```python
from build123d import *

# Parameters (mm, degrees)
EXTRUDE_1_DEPTH     = 9
EXTRUDE_2_DEPTH     = 13
SKETCH_5_R          = 4.25
CUT_EXTRUDE_1_DEPTH = 7


with BuildPart() as part:
    # Эскиз1 → Повернуть1 (revolve)
    with BuildSketch(Plane.XY, mode=Mode.PRIVATE) as revolve_1_sk:
        Polygon((0, 0), (-30, 0), (-30, 6), (-17, 6), (-16, 20), (-12, 20), (-12, 22), (-8, 26), (-8, 29), (-8, 38), (-8, 186), (-6, 188), (0, 188), align=None)
    revolve(revolve_1_sk.sketch.rotate(Axis((0, 0, 0), (0, 1, 0)), 180), axis=Axis((0, 0, 0), (0, 1, 0)))  # turned: the seam where the file's is

    # Эскиз2 → Бобышка-Вытянуть1 (add)
    with BuildSketch(Plane(origin=(0, 29, 0), x_dir=(1, 0, 0), z_dir=(0, 1, 0))):
        Polygon((0, 13.856406461), (-12, 6.92820323), (-12, -6.92820323), (0, -13.856406461), (12, -6.92820323), (12, 6.92820323), align=None)
    extrude(amount=EXTRUDE_1_DEPTH)

    # Эскиз3 → Бобышка-Вытянуть2 (add)
    with BuildSketch(Plane(origin=(0, 112, 0), x_dir=(1, 0, 0), z_dir=(0, 1, 0))):
        Polygon((12, 6.92820323), (0, 13.856406461), (-12, 6.92820323), (-12, -6.92820323), (0, -13.856406461), (12, -6.92820323), align=None)
    extrude(amount=EXTRUDE_2_DEPTH)

    # Эскиз4 → Вырез-Повернуть2 (revolve, cut)
    with BuildSketch(Plane.XY, mode=Mode.PRIVATE) as cut_revolve_2_sk:
        Polygon((-23.258330249, 125), (-12, 125), (-23.258330249, 118.5), align=None)
        Polygon((-23.258330249, 112), (-23.258330249, 118.5), (-12, 112), align=None)
        Polygon((-19.794228634, 38), (-19.794228634, 33.5), (-12, 38), align=None)
        Polygon((-19.794228634, 33.5), (-19.794228634, 29), (-12, 29), align=None)
    revolve(cut_revolve_2_sk.sketch.rotate(Axis((0, 188, 0), (0, -1, 0)), 180), axis=Axis((0, 188, 0), (0, -1, 0)), mode=Mode.SUBTRACT)  # turned: the seam where the file's is

    # Эскиз5 → Вырез-Вытянуть1 (cut, through all)
    with BuildSketch(Plane(origin=(0, 6, 0), x_dir=(1, 0, 0), z_dir=(0, 1, 0))):
        with Locations(Location((-23.75, 0, 0), (0, 0, 180))):  # turned: the seam where the file's is
            Circle(SKETCH_5_R)
        with Locations(Location((23.75, 0, 0), (0, 0, 180))):  # turned: the seam where the file's is
            Circle(SKETCH_5_R)
    extrude(amount=-CUT_EXTRUDE_1_DEPTH, mode=Mode.SUBTRACT)


solid = part.part
```
The model under review builds one solid part; all positions refer to its coordinate system, in mm. A direction names the side the tool comes from. Give positions to 0.01 mm unless a question says otherwise; leave off trailing zeros. Loops run counter-clockwise (first coordinate to the right, second up) from the corner with the lowest first, then second, coordinate; pieces in that order, holes last. Notation, with made-up numbers: (-33.75, 60) - (15.25, 60) arc R31 ccw to (15.25, 95) - close; hole circle Ø9 at (-27.5, 78). An arc over 180 degrees is marked (long way). Answer as a JSON object with one key per item and string values.
Q1. Insertion check: pin 1 (1.5 mm diameter, centred on x = 0, y = 113, fed in from -Z); pin 2 (10.5 mm diameter, centred on y = 115.5, z = -2.5, fed in from -X); pin 3 (10 mm diameter, centred on y = 119.5, z = -16.5, fed in from +X); pin 4 (7.5 mm diameter, centred on x = 23.75, z = 0, fed in from -Y). Each pin has a flat end and moves straight along its axis. Give the tip position at first contact, or say it passes through.
Worked out:
{"pin 1": "stops at z = -13.86", "pin 2": "stops at x = -12", "pin 3": "stops at x = 4.08", "pin 4": "passes through"}
Q2. Add section B-B on y = 122. State the section outline as (x, z) points, plus the area to 3 significant figures.
Worked out:
{"outline": "(-12, -6.93) - (0, -13.86) - (12, -6.93) - (12, 6.93) - (0, 13.86) - (-12, 6.93) - close", "area": "499 mm^2"}
Q3. Add section C-C on z = 19. State the section outline as (x, y) points, plus the area to 3 significant figures.
Worked out:
{"outline": "(-23.22, 0) - (23.22, 0) - (23.22, 6) - (-23.22, 6) - close", "area": "279 mm^2"}
Q4. Add section A-A on x = -23.75. State the section outline as (y, z) points, plus the area to 3 significant figures.
Worked out:
{"outline": "(0, -18.33) - (6, -18.33) - (6, -4.25) - (0, -4.25) - close; (0, 4.25) - (6, 4.25) - (6, 18.33) - (0, 18.33) - close", "area": "169 mm^2"}
Q5. For faces 4 (the flat face through (6.084, 33.437, -10.344)), 5 (the flat face through (12, 33, 0)), 6 (the conical face through (-0.03, 37.744, -12.443)), 7 (the cylindrical face through (-1.73, 74.48, 7.81)), list the 3-axis set-ups (+Z, -Z, +X, -X, +Y, -Y) from which the entire face can be reached by the end or side of a thin tool; tool diameter is ignored.
Worked out:
{"face 4": "-Z, +X, +Y", "face 5": "+Z, -Z, +X, +Y", "face 6": "-Z", "face 7": "none"}
Q6. To check wall thickness, follow line 1 along Y through (x, z) = (8, -1); line 2 along Y through (x, z) = (6.5, 7.5); line 3 along Y through (x, z) = (8, -20.5). State the ranges of each line that lie inside material, in increasing order.
Worked out:
{"line 1": "y = 0 to 25.94, 29 to 38, 112 to 125", "line 2": "y = 0 to 24.08, 29 to 38, 112 to 125", "line 3": "y = 0 to 6"}
Q7. Mouldability with a two-part tool opening along Y and no side actions: class faces 1 (the conical face through (-0.03, 124.74, -12.45)), 2 (the flat face through (12, 118, 0)), 3 (the conical face through (-10.8, 29.26, -6.2)) as +Y half, -Y half, draft (parallel to the pull), parting line (faces both ways), or undercut.
Worked out:
{"face 1": "+Y half", "face 2": "draft", "face 3": "undercut"}
Q8. Add section D-D on y = 94.5. State the section outline as (x, z) points, plus the area to 3 significant figures.
Worked out:
{"outline": "circle Ø16 at (0, 0)", "area": "201 mm^2"}
